The listing builds one solid part. Answer for the finished solid, in the listing's coordinates (mm). A direction names the side the tool comes from. Coordinates: 2 decimals unless noted, no trailing zeros. Order: outer loops, then holes, each group sorted by start corner. A loop starts at its lowest first (then second) coordinate and runs counter-clockwise, first axis right, second up. Notation, with made-up numbers: (76.25, 51) -> (95.25, 51) arc R30 cw to (95.25, 81) -> close; hole circle Ø8 at (-22, -17.5). An arc over 180 degrees is marked (long way). Write item = value, one per line.
from build123d import *

# Parameters (mm, degrees)
EXTRUDE_1_DEPTH     = 6
CUT_EXTRUDE_1_DEPTH = 4.5
EXTRUDE_4_DEPTH     = 3
SKETCH_4_R          = 1.6
CUT_EXTRUDE_2_DEPTH = 6
EXTRUDE_START       = 1.25
EXTRUDE_5_DEPTH     = 1.25
SKETCH_6_R          = 3
CUT_EXTRUDE_3_DEPTH = 1
FILLET_1_R          = 2


with BuildPart() as part:
    # Эскиз1 → Бобышка-Вытянуть1 (new body)
    with BuildSketch(Plane.XY):
        with BuildLine():
            Line((-17, -15), (17, -15))
            ThreePointArc((17, -15), (20.181980515, -13.681980515), (21.5, -10.5))
            Line((21.5, -10.5), (21.5, 10.5))
            ThreePointArc((21.5, 10.5), (20.181980515, 13.681980515), (17, 15))
            Line((17, 15), (-17, 15))
            ThreePointArc((-17, 15), (-20.181980515, 13.681980515), (-21.5, 10.5))
            Line((-21.5, 10.5), (-21.5, -10.5))
            ThreePointArc((-21.5, -10.5), (-20.181980515, -13.681980515), (-17, -15))
        make_face()
    extrude(amount=EXTRUDE_1_DEPTH)

    # Эскиз2 → Вырез-Вытянуть1 (cut)
    with BuildSketch(Plane.XY.offset(6)):
        with BuildLine():
            Line((-17, -12.75), (17, -12.75))
            ThreePointArc((17, -12.75), (18.590990258, -12.090990258), (19.25, -10.5))
            Line((19.25, -10.5), (19.25, 10.5))
            ThreePointArc((19.25, 10.5), (18.590990258, 12.090990258), (17, 12.75))
            Line((17, 12.75), (-17, 12.75))
            ThreePointArc((-17, 12.75), (-18.590990258, 12.090990258), (-19.25, 10.5))
            Line((-19.25, 10.5), (-19.25, -10.5))
            ThreePointArc((-19.25, -10.5), (-18.590990258, -12.090990258), (-17, -12.75))
        make_face()
    extrude(amount=-CUT_EXTRUDE_1_DEPTH, mode=Mode.SUBTRACT)

    # Эскиз3 → Бобышка-Вытянуть4 (add)
    with BuildSketch(Plane.XY.offset(1.5)):
        with BuildLine():
            Line((-13.5, 10), (-13.5, 13))
            Line((-13.5, 13), (-19.5, 13))
            Line((-19.5, 13), (-19.5, 7))
            Line((-19.5, 7), (-16.5, 7))
            ThreePointArc((-16.5, 7), (-14.378679656, 7.878679656), (-13.5, 10))
        make_face()
        with BuildLine():
            Line((-16.5, -7), (-19.5, -7))
            Line((-19.5, -7), (-19.5, -13))
            Line((-19.5, -13), (-13.5, -13))
            Line((-13.5, -13), (-13.5, -10))
            ThreePointArc((-13.5, -10), (-14.378679656, -7.878679656), (-16.5, -7))
        make_face()
        with BuildLine():
            Line((16.5, -7), (19.5, -7))
            Line((19.5, -7), (19.5, -13))
            Line((19.5, -13), (13.5, -13))
            Line((13.5, -13), (13.5, -10))
            ThreePointArc((13.5, -10), (14.378679656, -7.878679656), (16.5, -7))
        make_face()
        with BuildLine():
            Line((13.5, 10), (13.5, 13))
            Line((13.5, 13), (19.5, 13))
            Line((19.5, 13), (19.5, 7))
            Line((19.5, 7), (16.5, 7))
            ThreePointArc((16.5, 7), (14.378679656, 7.878679656), (13.5, 10))
        make_face()
    extrude(amount=EXTRUDE_4_DEPTH)

    # Эскиз4 → Вырез-Вытянуть2 (cut)
    with BuildSketch(Plane.XY.offset(4.5)):
        with Locations((16.5, -10)):
            Circle(SKETCH_4_R)
        with Locations((-16.5, -10)):
            Circle(SKETCH_4_R)
        with Locations((-16.5, 10)):
            Circle(SKETCH_4_R)
        with Locations((16.5, 10)):
            Circle(SKETCH_4_R)
    extrude(amount=-CUT_EXTRUDE_2_DEPTH, mode=Mode.SUBTRACT)

    # Эскиз5 → Бобышка-Вытянуть5 (add)
    with BuildSketch(Plane.XY.offset(6).offset(EXTRUDE_START)):
        with BuildLine():
            Line((17, -13.75), (-17, -13.75))
            ThreePointArc((-17, -13.75), (-19.298097039, -12.798097039), (-20.25, -10.5))
            Line((-20.25, -10.5), (-20.25, 10.5))
            ThreePointArc((-20.25, 10.5), (-19.298097039, 12.798097039), (-17, 13.75))
            Line((-17, 13.75), (17, 13.75))
            ThreePointArc((17, 13.75), (19.298097039, 12.798097039), (20.25, 10.5))
            Line((20.25, 10.5), (20.25, -10.5))
            ThreePointArc((20.25, -10.5), (19.298097039, -12.798097039), (17, -13.75))
        make_face()
        with BuildLine():
            Line((17, -12.75), (-17, -12.75))
            ThreePointArc((-17, -12.75), (-18.590990258, -12.090990258), (-19.25, -10.5))
            Line((-19.25, -10.5), (-19.25, 10.5))
            ThreePointArc((-19.25, 10.5), (-18.590990258, 12.090990258), (-17, 12.75))
            Line((-17, 12.75), (17, 12.75))
            ThreePointArc((17, 12.75), (18.590990258, 12.090990258), (19.25, 10.5))
            Line((19.25, 10.5), (19.25, -10.5))
            ThreePointArc((19.25, -10.5), (18.590990258, -12.090990258), (17, -12.75))
        make_face(mode=Mode.SUBTRACT)
    extrude(amount=-EXTRUDE_5_DEPTH)

    # Эскиз6 → Вырез-Вытянуть3 (cut)
    with BuildSketch(Plane(origin=(0, 0, 0), x_dir=(-1, 0, 0), z_dir=(0, 0, -1))):
        with Locations((16.5, -10)):
            Circle(SKETCH_6_R)
        with Locations((-16.5, -10)):
            Circle(SKETCH_6_R)
        with Locations((16.5, 10)):
            Circle(SKETCH_6_R)
        with Locations((-16.5, 10)):
            Circle(SKETCH_6_R)
    extrude(amount=-CUT_EXTRUDE_3_DEPTH, mode=Mode.SUBTRACT)

    # Скругление1
    fillet_1_edges = [part.edges().sort_by_distance(p)[0] for p in [
        (21.5, 0, 0),
        (20.181980515, -13.681980515, 0),
        (0, -15, 0),
        (-20.181980515, -13.681980515, 0),
        (-21.5, 0, 0),
        (-20.181980515, 13.681980515, 0),
        (0, 15, 0),
        (20.181980515, 13.681980515, 0),
    ]]
    fillet(fillet_1_edges, radius=FILLET_1_R - 0.0001)  # a hair under: the kernel refuses the full size


solid = part.part
Q1. Section D-D, the plane y = -6.25 is taken. Give the vertices of the cut face in (x, z), plus the area to 3 significant figures.
The answers:
outline = (-21.5, 2) arc R2 ccw to (-19.5, 0) -> (19.5, 0) arc R2 ccw to (21.5, 2) -> (21.5, 6) -> (20.25, 6) -> (20.25, 7.25) -> (19.25, 7.25) -> (19.25, 1.5) -> (-19.25, 1.5) -> (-19.25, 7.25) -> (-20.25, 7.25) -> (-20.25, 6) -> (-21.5, 6) -> close
area = 85.5 mm2
Q2. Section A-A, the plane z = 2.5 is taken. Give the vertices of the cut face in (x, y).
The answers:
outline = (-21.5, -10.5) arc R4.5 ccw to (-17, -15) -> (17, -15) arc R4.5 ccw to (21.5, -10.5) -> (21.5, 10.5) arc R4.5 ccw to (17, 15) -> (-17, 15) arc R4.5 ccw to (-21.5, 10.5) -> close; hole (-19.25, -7) -> (-16.5, -7) arc R3 cw to (-13.5, -10) -> (-13.5, -12.75) -> (13.5, -12.75) -> (13.5, -10) arc R3 cw to (16.5, -7) -> (19.25, -7) -> (19.25, 7) -> (16.5, 7) arc R3 cw to (13.5, 10) -> (13.5, 12.75) -> (-13.5, 12.75) -> (-13.5, 10) arc R3 cw to (-16.5, 7) -> (-19.25, 7) -> close; hole circle Ø3.2 at (-16.5, -10); hole circle Ø3.2 at (-16.5, 10); hole circle Ø3.2 at (16.5, -10); hole circle Ø3.2 at (16.5, 10)
Q3. Section C-C, the plane z = 5.25 is taken. Give the vertices of the cut face in (x, y), plus the area to 3 significant figures.
The answers:
outline = (-21.5, -10.5) arc R4.5 ccw to (-17, -15) -> (17, -15) arc R4.5 ccw to (21.5, -10.5) -> (21.5, 10.5) arc R4.5 ccw to (17, 15) -> (-17, 15) arc R4.5 ccw to (-21.5, 10.5) -> close; hole (-19.25, -10.5) arc R2.25 ccw to (-17, -12.75) -> (17, -12.75) arc R2.25 ccw to (19.25, -10.5) -> (19.25, 10.5) arc R2.25 ccw to (17, 12.75) -> (-17, 12.75) arc R2.25 ccw to (-19.25, 10.5) -> close
area = 295 mm2
Q4. The mould has two halves that part along Y. Classify faces 1 (the face through (0, 0, 0)), 2 (the face through (-14.4, 7.86, 2.98)), 3 (the face through (-0.24, 14.43, 0.6)): released by +Y, released by -Y, zero draft, split by the parting line, or undercut.
The answers:
face_1 = zero draft
face_2 = undercut
face_3 = released by +Y
Q5. A tool of negligible diameter and unlimited length cuts with its end or side. For faces 4 (the face through (20.25, 0, 7)), 5 (the face through (-13.5, -11, 3)), 6 (the face through (-18, -11, 1)), 7 (the face through (0, 13.75, 7)), from which of +Z, -Z, +X, -X, +Y, -Y can it reach the whole face along a straight path? Write none if from no direction.
The answers:
face_4 = +Z, +X, +Y, -Y
face_5 = +Z
face_6 = -Z
face_7 = +Z, +X, -X, +Y
Q6. Find the intervals of material crossed by line 1 along Y through (x, z) = (16.5, 2.7); line 2 along Y through (x, z) = (-18.5, 0.5); line 3 along Y through (x, z) = (7.5, 3.25), in increasing order.
The answers:
line_1 = -15 to -11.6, -8.4 to -7, 7 to 8.4, 11.6 to 15
line_2 = -14.02 to -12.24, -7.76 to 7.76, 12.24 to 14.02
line_3 = -15 to -12.75, 12.75 to 15
Q7. Section B-B, the plane x = -16 is taken. Give the number of separate pieces and of enclosed holes in the cut face, plus the area to 3 significant figures.
The answers:
separate_pieces = 3
enclosed_holes = 0
area = 67.2 mm2
Q8. Each of these flat-tipped pins is pushed along its axis until it touches: pin 1 Ø1.4 at (y, z) = (11.5, 3) entering from +X; pin 2 Ø2 at (x, y) = (16.5, 10.5) entering from +Z; pin 3 Ø5.5 at (x, y) = (-16.5, -10) entering from -Z; pin 4 Ø2 at (x, y) = (14, 8.5) entering from +Z. Where does it stop, or does it pass through?
The answers:
pin_1 = 21.49
pin_2 = through
pin_3 = 1
pin_4 = 4.5
